Geometry check sheet. Reference: the model listing, model coordinates, mm. A direction names the side the tool comes from. Coordinates: 2 decimals unless noted, no trailing zeros. Write each loop counter-clockwise with the first axis right and the second up, starting at its lowest first coordinate (ties: lowest second). Pieces come first, ordered by that corner, then holes. Notation, with made-up numbers: (-16, 9) -> (22, 9) arc R16 ccw to (22, 30) -> close; hole circle Ø8 at (17.25, 89). An arc over 180 degrees is marked (long way). Use a Markdown table: item, result.
```python
from build123d import *
from build123d.topology import SkipClean

# Parameters (mm, degrees)
SKETCH1_R           = 19
SKETCH1_R_2         = 2.11
BOSS_EXTRUDE1_DEPTH = 10.5
BOSS_EXTRUDE2_DEPTH = 1
CIRPATTERN1_COUNT   = 4
SKETCH4_R           = 7.5
BOSS_EXTRUDE3_DEPTH = 9.5
EXTRUDE_THIN1_DEPTH = 17
CIRPATTERN2_COUNT   = 3
CUT_EXTRUDE1_DEPTH  = 3.7
CIRPATTERN3_COUNT   = 4


with BuildPart() as part:
    # Sketch1 → Boss-Extrude1 (new body)
    with BuildSketch(Plane.XY):
        with BuildLine():
            Line((-16, 20), (16, 20))
            ThreePointArc((16, 20), (18.828427125, 18.828427125), (20, 16))
            Line((20, 16), (20, -16))
            ThreePointArc((20, -16), (18.828427125, -18.828427125), (16, -20))
            Line((16, -20), (-16, -20))
            ThreePointArc((-16, -20), (-18.828427125, -18.828427125), (-20, -16))
            Line((-20, -16), (-20, 16))
            ThreePointArc((-20, 16), (-18.828427125, 18.828427125), (-16, 20))
        make_face()
        Circle(SKETCH1_R, mode=Mode.SUBTRACT)
        with Locations((-16, 16)):
            Circle(SKETCH1_R_2, mode=Mode.SUBTRACT)
        with Locations((-16, -16)):
            Circle(SKETCH1_R_2, mode=Mode.SUBTRACT)
        with Locations((16, -16)):
            Circle(SKETCH1_R_2, mode=Mode.SUBTRACT)
        with Locations((16, 16)):
            Circle(SKETCH1_R_2, mode=Mode.SUBTRACT)
    extrude(amount=BOSS_EXTRUDE1_DEPTH)

    # Sketch2 → Boss-Extrude2 (add)
    with BuildSketch(Plane.XY.offset(10.5)):
        with BuildLine():
            Line((-1.25, 17.85882135), (-1.25, 8.196798155))
            ThreePointArc((-1.25, 8.196798155), (-1.454793774, 7.590459093), (-1.985294118, 7.232468961))
            ThreePointArc((-1.985294118, 7.232468961), (0, -7.5), (1.985294118, 7.232468961))
            ThreePointArc((1.985294118, 7.232468961), (1.454793774, 7.590459093), (1.25, 8.196798155))
            Line((1.25, 8.196798155), (1.25, 17.85882135))
            ThreePointArc((1.25, 17.85882135), (1.588562172, 18.60882135), (2.375, 18.850978091))
            ThreePointArc((2.375, 18.850978091), (0, 19), (-2.375, 18.850978091))
            ThreePointArc((-2.375, 18.850978091), (-1.588562172, 18.60882135), (-1.25, 17.85882135))
        make_face()
    boss_extrude2 = extrude(amount=-BOSS_EXTRUDE2_DEPTH)

    # CirPattern1: Boss-Extrude2 ×4 about axis
    cirpattern1_axis = Axis((0, 0, 0), (0, 0, 1))
    for i in range(1, CIRPATTERN1_COUNT):
        add(boss_extrude2.rotate(cirpattern1_axis, i * 360 / CIRPATTERN1_COUNT))

    # Sketch4 → Boss-Extrude3 (add)
    with SkipClean():  # keep this step's faces unmerged: merging them makes the solid invalid here
        with BuildSketch(Plane(origin=(0, 0, 9.5), x_dir=(-1, 0, 0), z_dir=(0, 0, -1))):
            with Locations(Location((0, 0, 0), (0, 0, 164.650522983))):  # turned: the seam where the file's is
                Circle(SKETCH4_R)
        extrude(amount=BOSS_EXTRUDE3_DEPTH)

    # Sketch5 → Extrude-Thin1 (add)
    with SkipClean():  # keep this step's faces unmerged: merging them makes the solid invalid here
        with BuildSketch(Plane(origin=(0, 0, 0), x_dir=(1, 0, 0), z_dir=(0, 1, 0))):
            with BuildLine():
                ThreePointArc((-6.073641938, -8.543547558), (-0.600270019, -4.001821599), (6.131264125, -1.705841866))
                Line((6.131264125, -1.705841866), (6.423685209, -3.684348857))
                ThreePointArc((6.423685209, -3.684348857), (0.377258659, -5.746653305), (-4.539056193, -9.826141254))
                Line((-4.539056193, -9.826141254), (-6.073641938, -8.543547558))
            make_face()
        extrude_thin1 = extrude(amount=EXTRUDE_THIN1_DEPTH)

    # CirPattern2: Extrude-Thin1 ×3 about axis
    with SkipClean():  # keep this step's faces unmerged: merging them makes the solid invalid here
        cirpattern2_axis = Axis((0, 0, 0), (0, 0, 1))
        for i in range(1, CIRPATTERN2_COUNT):
            add(extrude_thin1.rotate(cirpattern2_axis, i * 360 / CIRPATTERN2_COUNT))

    # Sketch6 → Cut-Extrude1 (cut)
    with SkipClean():  # keep this step's faces unmerged: merging them makes the solid invalid here
        with BuildSketch(Plane(origin=(0, 0, 0), x_dir=(-1, 0, 0), z_dir=(0, 0, -1))):
            Polygon((-16.896575472, 19.346065215), (-19.346065215, 16.896575472), (-18.449489743, 13.550510257), (-15.103424528, 12.653934785), (-12.653934785, 15.103424528), (-13.550510257, 18.449489743), align=None)
        cut_extrude1 = extrude(amount=-CUT_EXTRUDE1_DEPTH, mode=Mode.SUBTRACT)

    # CirPattern3: Cut-Extrude1 ×4 about axis
    with SkipClean():  # keep this step's faces unmerged: merging them makes the solid invalid here
        cirpattern3_axis = Axis((0, 0, 0), (0, 0, 1))
        for i in range(1, CIRPATTERN3_COUNT):
            add(cut_extrude1.rotate(cirpattern3_axis, i * 360 / CIRPATTERN3_COUNT), mode=Mode.SUBTRACT)


solid = part.part
```
Item 1: Tool access check on faces 5 (the cylindrical face through (0.46, 11.8, 5.7)), 6 (the flat face through (-1.25, 13, 10)), 7 (the cylindrical face through (18.62, 1.6, 10.01)), 8 (the flat face through (5.8, -10.6, 2.7)). Record the directions out of +Z, -Z, +X, -X, +Y, -Y that give a thin tool (end or side, any length) a straight path to the whole face; none if there is none.
Answer block:
| item | result |
|---|---|
| face 5 | none |
| face 6 | +Z |
| face 7 | +Z, -Z |
| face 8 | -Z |
Item 2: Mould release check, pull along X, two halves, no side actions. Record for faces 1 (the flat face through (16.753, -13.096, 1.824)), 2 (the cylindrical face through (18.797, 18.859, 5.176)), 3 (the flat face through (-20, 0, 5)), 4 (the flat face through (-13.11, 16.8, 1.82)): +X half, -X half, draft (parallel to the pull), parting line (faces both ways), or undercut.
Answer block:
| item | result |
|---|---|
| face 1 | undercut |
| face 2 | +X half |
| face 3 | -X half |
| face 4 | undercut |
Item 3: Depth check by flat-ended pin: P1, Ø2, axis at x = -14.5, y = -17.5, coming from the -Z side; P2, Ø2.5, axis at x = 16, y = -16, coming from the -Z side; P3, Ø4, axis at x = -11.5, y = 1, coming from the -Z side; P4, Ø1.4, axis at x = -0.5, y = -11.5, coming from the -Z side. Enter the tip coordinate at first touch or a pass-through.
Answer block:
| item | result |
|---|---|
| P1 | stops at z = 3.7 |
| P2 | passes through |
| P3 | stops at z = 1.71 |
| P4 | stops at z = 9.5 |
Item 4: Section check A-A on z = 1. Count the separate pieces of the cut face and the enclosed holes in it, then the cut area to 3 significant figures.
Answer block:
| item | result |
|---|---|
| separate pieces | 2 |
| enclosed holes | 5 |
| area | 504 mm^2 |
Item 5: Thickness scan on L1, parallel to Y at x = 0, z = 8.25; L2, parallel to X at y = 16, z = 8. Record the ranges inside material, lowest first. Write a range as [from, to].
Answer block:
| item | result |
|---|---|
| L1 | y = [-20, -19], [-7.5, 7.5], [19, 20] |
| L2 | x = [-20, -18.11], [-13.89, -10.25], [-5.6, -2.77], [10.25, 13.89], [18.11, 20] |
Item 6: Section check B-B on z = 6.75. Record the boundary of the cut face in (x, y).
Answer block:
| item | result |
|---|---|
| outline | (-20, -16) arc R4 ccw to (-16, -20) -> (16, -20) arc R4 ccw to (20, -16) -> (20, 16) arc R4 ccw to (16, 20) -> (-16, 20) arc R4 ccw to (-20, 16) -> close; (-14.12, -9.55) -> (-12.54, -12.29) -> (-3.09, -6.83) arc R7.5 ccw to (7.01, -2.65) -> (15.33, -7.45) -> (16.91, -4.71) -> (7.46, 0.74) arc R7.5 ccw to (-1.21, 7.4) -> (-1.21, 17) -> (-4.37, 17) -> (-4.37, 6.09) arc R7.5 ccw to (-5.81, -4.75) -> close; hole circle Ø38 at (0, 0); hole circle Ø4.22 at (-16, -16); hole circle Ø4.22 at (-16, 16); hole circle Ø4.22 at (16, -16); hole circle Ø4.22 at (16, 16) |
